from build123d import *

# Parameters (mm, degrees)
SKETCH1_W                     = 26.6
SKETCH1_H                     = 19.5
BASE_DEPTH                    = 8.5
SKETCH2_R                     = 2.5
BOSS_EXTRUDE2_DEPTH           = 0.25
BOSS_EXTRUDE2_DRAFT           = 40
SKETCH2_W                     = 9.7
SKETCH2_H                     = 8.8
BOSS_EXTRUDE2_PROFILE_2_DEPTH = 0.25
BOSS_EXTRUDE2_PROFILE_2_DRAFT = 40
SKETCH3_W                     = 8.480450184
SKETCH3_H                     = 7.580450184
CUT_EXTRUDE1_DEPTH            = 0.25
SKETCH4_W                     = 10
SKETCH4_H                     = 8.5
BOSS_EXTRUDE3_DEPTH           = 0.25
BOSS_EXTRUDE3_TAPER           = 40
SKETCH5_W                     = 8.980450184
SKETCH5_H                     = 7.480450184
CUT_EXTRUDE2_DEPTH            = 0.25
FILLET1_R                     = 1
SKETCH6_W                     = 6.5
SKETCH6_H                     = 2.5
CONNECTOR1_DEPTH              = 0.2
SKETCH7_W                     = 4.5
SKETCH7_H                     = 2.2
CONNECTOR2_DEPTH              = 0.25
SKETCH8_W                     = 3.3
SKETCH8_H                     = 13
SKETCH8_W_2                   = 2.8
SKETCH8_H_2                   = 14.25
PCB_DEPTH                     = 0.9
CUT_EXTRUDE3_REACH            = 23.263
SKETCH9_R                     = 0.325


with BuildPart() as part:
    # Sketch1 → Base (new body)
    with BuildSketch(Plane.XY):
        Rectangle(SKETCH1_W, SKETCH1_H)
    extrude(amount=BASE_DEPTH)


with BuildPart() as boss_extrude2_tool:
    # Sketch2 → Boss-Extrude2 (with draft: the straight prism first)
    with BuildSketch(Plane.XY.offset(8.5)):
        with Locations((7.8, -4.75)):
            Circle(SKETCH2_R)
    extrude(amount=BOSS_EXTRUDE2_DEPTH)
    # Boss-Extrude2: the draft: its side faces are tilted about the plane it starts from
    boss_extrude2_sides = [boss_extrude2_tool.faces().sort_by_distance(p)[0] for p in [
        (5.3, -4.75, 8.625),
    ]]
    draft(boss_extrude2_sides, Plane.XY.offset(8.5), BOSS_EXTRUDE2_DRAFT)


with BuildPart() as part_1:
    add(part.part)

    # Boss-Extrude2: add boss_extrude2_tool
    add(boss_extrude2_tool.part)


with BuildPart() as boss_extrude2_profile_2_tool:
    # Sketch2 → Boss-Extrude2 profile 2 (with draft: the straight prism first)
    with BuildSketch(Plane.XY.offset(8.5)):
        with Locations((8.45, 4.35)):
            Rectangle(SKETCH2_W, SKETCH2_H)
    extrude(amount=BOSS_EXTRUDE2_PROFILE_2_DEPTH)
    # Boss-Extrude2 profile 2: the draft: its side faces are tilted about the plane it starts from
    boss_extrude2_profile_2_sides = [boss_extrude2_profile_2_tool.faces().sort_by_distance(p)[0] for p in [
        (3.6, 4.35, 8.625),
        (8.45, -0.05, 8.625),
        (13.3, 4.35, 8.625),
        (8.45, 8.75, 8.625),
    ]]
    draft(boss_extrude2_profile_2_sides, Plane.XY.offset(8.5), BOSS_EXTRUDE2_PROFILE_2_DRAFT)


with BuildPart() as part_2:
    add(part_1.part)

    # Boss-Extrude2 profile 2: add boss_extrude2_profile_2_tool
    add(boss_extrude2_profile_2_tool.part)

    # Sketch3 → Cut-Extrude1 (cut)
    with BuildSketch(Plane.XY.offset(8.75)):
        with Locations((8.45, 4.35)):
            Rectangle(SKETCH3_W, SKETCH3_H)
    extrude(amount=-CUT_EXTRUDE1_DEPTH, mode=Mode.SUBTRACT)

    # Sketch4 → Boss-Extrude3 (add)
    with BuildSketch(Plane.XZ.offset(9.75)):
        with Locations((-4.3, 4.25)):
            Rectangle(SKETCH4_W, SKETCH4_H)
    extrude(amount=BOSS_EXTRUDE3_DEPTH, taper=BOSS_EXTRUDE3_TAPER)

    # Sketch5 → Cut-Extrude2 (cut)
    with BuildSketch(Plane.XZ.offset(10)):
        with Locations((-4.3, 4.25)):
            Rectangle(SKETCH5_W, SKETCH5_H)
    extrude(amount=-CUT_EXTRUDE2_DEPTH, mode=Mode.SUBTRACT)

    # Fillet1
    fillet1_edges = [part_2.edges().sort_by_distance(p)[0] for p in [
        (-13.3, 9.75, 4.25),
        (13.3, 9.75, 4.25),
        (13.3, -9.75, 4.25),
        (-13.3, -9.75, 4.25),
    ]]
    fillet(fillet1_edges, radius=FILLET1_R)

    # Sketch6 → Connector1 (add)
    with BuildSketch(Plane(origin=(0, 0, 0), x_dir=(-1, 0, 0), z_dir=(0, 0, -1))):
        with Locations((0.95, 4.8)):
            Rectangle(SKETCH6_W, SKETCH6_H)
    extrude(amount=CONNECTOR1_DEPTH)

    # Sketch7 → Connector2 (add)
    with BuildSketch(Plane(origin=(0, 0, -0.2), x_dir=(-1, 0, 0), z_dir=(0, 0, -1))):
        with Locations((0.95, 4.8)):
            Rectangle(SKETCH7_W, SKETCH7_H)
    extrude(amount=CONNECTOR2_DEPTH)

    # Sketch8 → PCB (add)
    with BuildSketch(Plane(origin=(0, 0, 0), x_dir=(-1, 0, 0), z_dir=(0, 0, -1))):
        with Locations((14.95, -1.25)):
            Rectangle(SKETCH8_W, SKETCH8_H)
        with Locations((-14.7, 0.075)):
            Rectangle(SKETCH8_W_2, SKETCH8_H_2)
    extrude(amount=-PCB_DEPTH)

    # Sketch9 → Cut-Extrude3 (cut, up to next)
    with BuildSketch(Plane(origin=(0, 0, 0), x_dir=(-1, 0, 0), z_dir=(0, 0, -1)), mode=Mode.PRIVATE) as cut_extrude3_sk1:
        with Locations((15.1, -5.05)):
            Circle(SKETCH9_R)
    cut_extrude3_tool1 = extrude(cut_extrude3_sk1.sketch, amount=-CUT_EXTRUDE3_REACH, mode=Mode.PRIVATE) & part_2.part
    # Sketch9 → Cut-Extrude3 (cut, up to next)
    with BuildSketch(Plane(origin=(0, 0, 0), x_dir=(-1, 0, 0), z_dir=(0, 0, -1)), mode=Mode.PRIVATE) as cut_extrude3_sk2:
        with Locations((15.1, -2.51)):
            Circle(SKETCH9_R)
    cut_extrude3_tool2 = extrude(cut_extrude3_sk2.sketch, amount=-CUT_EXTRUDE3_REACH, mode=Mode.PRIVATE) & part_2.part
    # Sketch9 → Cut-Extrude3 (cut, up to next)
    with BuildSketch(Plane(origin=(0, 0, 0), x_dir=(-1, 0, 0), z_dir=(0, 0, -1)), mode=Mode.PRIVATE) as cut_extrude3_sk3:
        with Locations((15.1, 0.03)):
            Circle(SKETCH9_R)
    cut_extrude3_tool3 = extrude(cut_extrude3_sk3.sketch, amount=-CUT_EXTRUDE3_REACH, mode=Mode.PRIVATE) & part_2.part
    # Sketch9 → Cut-Extrude3 (cut, up to next)
    with BuildSketch(Plane(origin=(0, 0, 0), x_dir=(-1, 0, 0), z_dir=(0, 0, -1)), mode=Mode.PRIVATE) as cut_extrude3_sk4:
        with Locations((15.1, 2.57)):
            Circle(SKETCH9_R)
    cut_extrude3_tool4 = extrude(cut_extrude3_sk4.sketch, amount=-CUT_EXTRUDE3_REACH, mode=Mode.PRIVATE) & part_2.part
    # Sketch9 → Cut-Extrude3 (cut, up to next)
    with BuildSketch(Plane(origin=(0, 0, 0), x_dir=(-1, 0, 0), z_dir=(0, 0, -1)), mode=Mode.PRIVATE) as cut_extrude3_sk5:
        with Locations((-14.44, -5)):
            Circle(SKETCH9_R)
    cut_extrude3_tool5 = extrude(cut_extrude3_sk5.sketch, amount=-CUT_EXTRUDE3_REACH, mode=Mode.PRIVATE) & part_2.part
    # Sketch9 → Cut-Extrude3 (cut, up to next)
    with BuildSketch(Plane(origin=(0, 0, 0), x_dir=(-1, 0, 0), z_dir=(0, 0, -1)), mode=Mode.PRIVATE) as cut_extrude3_sk6:
        with Locations((-14.44, -2.46)):
            Circle(SKETCH9_R)
    cut_extrude3_tool6 = extrude(cut_extrude3_sk6.sketch, amount=-CUT_EXTRUDE3_REACH, mode=Mode.PRIVATE) & part_2.part
    # Sketch9 → Cut-Extrude3 (cut, up to next)
    with BuildSketch(Plane(origin=(0, 0, 0), x_dir=(-1, 0, 0), z_dir=(0, 0, -1)), mode=Mode.PRIVATE) as cut_extrude3_sk7:
        with Locations((-14.44, 0.08)):
            Circle(SKETCH9_R)
    cut_extrude3_tool7 = extrude(cut_extrude3_sk7.sketch, amount=-CUT_EXTRUDE3_REACH, mode=Mode.PRIVATE) & part_2.part
    # Sketch9 → Cut-Extrude3 (cut, up to next)
    with BuildSketch(Plane(origin=(0, 0, 0), x_dir=(-1, 0, 0), z_dir=(0, 0, -1)), mode=Mode.PRIVATE) as cut_extrude3_sk8:
        with Locations((-14.44, 2.62)):
            Circle(SKETCH9_R)
    cut_extrude3_tool8 = extrude(cut_extrude3_sk8.sketch, amount=-CUT_EXTRUDE3_REACH, mode=Mode.PRIVATE) & part_2.part
    # Sketch9 → Cut-Extrude3 (cut, up to next)
    with BuildSketch(Plane(origin=(0, 0, 0), x_dir=(-1, 0, 0), z_dir=(0, 0, -1)), mode=Mode.PRIVATE) as cut_extrude3_sk9:
        with Locations((-14.44, 5.16)):
            Circle(SKETCH9_R)
    cut_extrude3_tool9 = extrude(cut_extrude3_sk9.sketch, amount=-CUT_EXTRUDE3_REACH, mode=Mode.PRIVATE) & part_2.part
    add(cut_extrude3_tool1.solids().sort_by_distance((-15.1, -5.05, 0))[0], mode=Mode.SUBTRACT)
    add(cut_extrude3_tool2.solids().sort_by_distance((-15.1, -2.51, 0))[0], mode=Mode.SUBTRACT)
    add(cut_extrude3_tool3.solids().sort_by_distance((-15.1, 0.03, 0))[0], mode=Mode.SUBTRACT)
    add(cut_extrude3_tool4.solids().sort_by_distance((-15.1, 2.57, 0))[0], mode=Mode.SUBTRACT)
    add(cut_extrude3_tool5.solids().sort_by_distance((14.44, -5, 0))[0], mode=Mode.SUBTRACT)
    add(cut_extrude3_tool6.solids().sort_by_distance((14.44, -2.46, 0))[0], mode=Mode.SUBTRACT)
    add(cut_extrude3_tool7.solids().sort_by_distance((14.44, 0.08, 0))[0], mode=Mode.SUBTRACT)
    add(cut_extrude3_tool8.solids().sort_by_distance((14.44, 2.62, 0))[0], mode=Mode.SUBTRACT)
    add(cut_extrude3_tool9.solids().sort_by_distance((14.44, 5.16, 0))[0], mode=Mode.SUBTRACT)


solid = part_2.part
CAD build for the part. Positions are in the model's coordinates, mm. A direction names the side the tool comes from. Give positions to 0.01 mm unless a question says otherwise; leave off trailing zeros. Write each loop counter-clockwise with the first axis right and the second up, starting at its lowest first coordinate (ties: lowest second). Pieces come first, ordered by that corner, then holes. Notation, with made-up numbers: (88, -22) -> (119, -22) arc R17 cw to (119, 3) -> close; hole circle Ø6 at (21.25, 62). An arc over 180 degrees is marked (long way). Return JSON: item names as keys, results as strings.
Item 1: Band-saw the part on C-C (y = -1.75). List the corners of the cut face in (x, z), then the cut area to 3 significant figures.
Answer below:
{"outline": "(-16.6, 0) -> (16.1, 0) -> (16.1, 0.9) -> (13.3, 0.9) -> (13.3, 8.5) -> (-13.3, 8.5) -> (-13.3, 0.9) -> (-16.6, 0.9) -> close", "area": "232 mm2"}
Item 2: Band-saw the part on A-A (x = 14.44). List the corners of the cut face in (y, z) (3 decimals).
Answer below:
{"outline": "(-7.05, 0) -> (-5.325, 0) -> (-5.325, 0.9) -> (-7.05, 0.9) -> close; (-4.675, 0) -> (-2.785, 0) -> (-2.785, 0.9) -> (-4.675, 0.9) -> close; (-2.135, 0) -> (-0.245, 0) -> (-0.245, 0.9) -> (-2.135, 0.9) -> close; (0.405, 0) -> (2.295, 0) -> (2.295, 0.9) -> (0.405, 0.9) -> close; (2.945, 0) -> (4.835, 0) -> (4.835, 0.9) -> (2.945, 0.9) -> close; (5.485, 0) -> (7.2, 0) -> (7.2, 0.9) -> (5.485, 0.9) -> close"}
Item 3: Drill centre lines: probe 1 along Y at (x, z) = (14.44, 0.2) (3 decimals); probe 2 along Y at (x, z) = (-15.1, 0.35) (3 decimals); probe 3 along Z at (x, y) = (-11, 8.5). Where is each one in solid material? Low to high.
Answer below:
{"probe 1": "y = -7.05 to -5.325, -4.675 to -2.785, -2.135 to -0.245, 0.405 to 2.295, 2.945 to 4.835, 5.485 to 7.2", "probe 2": "y = -7.75 to -5.375, -4.725 to -2.835, -2.185 to -0.295, 0.355 to 2.245, 2.895 to 5.25", "probe 3": "z = 0 to 8.5"}
Item 4: Tool access for faces 1 (the flat face through (8, 4, 8.5)), 2 (the flat face through (14.7, 7.2, 0.4)), 3 (the flat face through (-14.9, -7.75, 0.4)): list every direction of +Z, -Z, +X, -X, +Y, -Y with a clear straight run to the whole face (end or side of a thin tool).
Answer below:
{"face 1": "+Z", "face 2": "+Z, -Z, +X, +Y", "face 3": "+Z, -Z, -X, -Y"}
Item 5: Drop flat-ended pins along their axis: pin 1 (6 mm diameter, centred on x = 8.5, y = 4.5, fed in from +Z); pin 2 (2 mm diameter, centred on y = -7, z = 4, fed in from -X); pin 3 (1.5 mm diameter, centred on y = -4.5, z = 6, fed in from +X); pin 4 (3.5 mm diameter, centred on x = -10.5, z = 3, fed in from -Y). Give the stop position or say it passes through.
Answer below:
{"pin 1": "stops at z = 8.5", "pin 2": "stops at x = -13.3", "pin 3": "stops at x = 13.3", "pin 4": "stops at y = -10"}
Item 6: Band-saw the part on B-B (x = -15.1). List the corners of the cut face in (y, z) (3 decimals).
Answer below:
{"outline": "(-7.75, 0) -> (-5.375, 0) -> (-5.375, 0.9) -> (-7.75, 0.9) -> close; (-4.725, 0) -> (-2.835, 0) -> (-2.835, 0.9) -> (-4.725, 0.9) -> close; (-2.185, 0) -> (-0.295, 0) -> (-0.295, 0.9) -> (-2.185, 0.9) -> close; (0.355, 0) -> (2.245, 0) -> (2.245, 0.9) -> (0.355, 0.9) -> close; (2.895, 0) -> (5.25, 0) -> (5.25, 0.9) -> (2.895, 0.9) -> close"}
